Source: CAD feature listing. Evaluate the final solid. Frame: model axes, mm. A direction names the side the tool comes from. Round coordinates to 2 decimals unless told otherwise and drop trailing zeros. Write each loop counter-clockwise with the first axis right and the second up, starting at its lowest first coordinate (ties: lowest second). Pieces come first, ordered by that corner, then holes.
from build123d import *

# Parameters (mm, degrees)
SKETCH1_W           = 40
SKETCH1_H           = 50
BOSS_EXTRUDE1_DEPTH = 10
SKETCH3_W           = 60
SKETCH3_H           = 10
BOSS_EXTRUDE2_DEPTH = 20
FILLET1_R           = 10
SKETCH4_R           = 19.5
SKETCH4_R_2         = 15
BOSS_EXTRUDE3_DEPTH = 20
SKETCH5_R           = 6.5
CUT_EXTRUDE1_DEPTH  = 100


with BuildPart() as part:
    # Sketch1 → Boss-Extrude1 (new body)
    with BuildSketch(Plane.XY):
        Rectangle(SKETCH1_W, SKETCH1_H)
    extrude(amount=BOSS_EXTRUDE1_DEPTH)

    # Sketch3 → Boss-Extrude2 (add, symmetric)
    with BuildSketch(Plane(origin=(0, 0, 0), x_dir=(0, 0, -1), z_dir=(1, 0, 0))):
        with Locations((20, -30)):
            Rectangle(SKETCH3_W, SKETCH3_H)
        with Locations((20, 30)):
            Rectangle(SKETCH3_W, SKETCH3_H)
    extrude(amount=BOSS_EXTRUDE2_DEPTH, both=True)

    # Fillet1
    fillet1_edges = [part.edges().sort_by_distance(p)[0] for p in [
        (0, -35, 10),
        (-20, -30, -50),
        (20, -30, -50),
        (0, 35, 10),
        (-20, 30, -50),
        (20, 30, -50),
    ]]
    fillet(fillet1_edges, radius=FILLET1_R)

    # Sketch4 → Boss-Extrude3 (add)
    with BuildSketch(Plane.XY.offset(10)):
        Circle(SKETCH4_R)
        Circle(SKETCH4_R_2, mode=Mode.SUBTRACT)
    extrude(amount=BOSS_EXTRUDE3_DEPTH)

    # Sketch5 → Cut-Extrude1 (cut)
    with BuildSketch(Plane.XZ.offset(35)):
        with Locations(Location((0, -40, 0), (0, 0, 270))):
            Circle(SKETCH5_R)
    extrude(amount=-CUT_EXTRUDE1_DEPTH, mode=Mode.SUBTRACT)


solid = part.part
1) Section query D-D on x = 16. Return the cut outline in (y, z), then the cut area to 3 significant figures.
Taken from the geometry:
outline: (-35, -48) - (-25, -48) - (-25, 0) - (25, 0) - (25, -48) - (35, -48) - (35, 0) arc R10 ccw to (25, 10) - (11.15, 10) - (11.15, 30) - (-11.15, 30) - (-11.15, 10) - (-25, 10) arc R10 ccw to (-35, 0) - close
area: 2,060 mm2
2) Pull-direction query (X, two-part tool) for faces 4 (the face through (-16.99, 30.07, -47.15)), 5 (the face through (0, -25, -25)), 6 (the face through (0.286, -30.07, -33.506)); classes: released by +X, released by -X, zero draft, split by the parting line, or undercut.
Taken from the geometry:
face 4: released by -X
face 5: zero draft
face 6: undercut
3) Contact query for flat-ended pins moving along their axis: P1, Ø1, axis at x = 1, y = 13, coming from the -Z side; P2, Ø12, axis at x = 6.5, y = -1.5, coming from the +Z side; P3, Ø8, axis at y = -12, z = 22, coming from the -X side. Output: stop coordinate, or through.
Taken from the geometry:
P1: stops at z = 0
P2: stops at z = 10
P3: stops at x = -17.78
4) Section query C-C on y = -4. Return the cut outline in (x, z), then the cut area to 3 significant figures.
Taken from the geometry:
outline: (-20, 0) - (20, 0) - (20, 10) - (19.09, 10) - (19.09, 30) - (14.46, 30) - (14.46, 10) - (-14.46, 10) - (-14.46, 30) - (-19.09, 30) - (-19.09, 10) - (-20, 10) - close
area: 585 mm2
5) Material intervals for line 1 (X direction, y = -32, z = -40); line 2 (Y direction, x = 6.5, z = -43.5); line 3 (Y direction, x = 0, z = 24), sorted ascending.
Taken from the geometry:
line 1: x = -20 to -6.5, 6.5 to 20
line 2: y = -35 to -25, 25 to 35
line 3: y = -19.5 to -15, 15 to 19.5
6) Reachability of faces 1 (the face through (20, 0, 2)), 2 (the face through (0, 0, 0)), 3 (the face through (-2.539, 19.334, 19.86)) from +Z, -Z, +X, -X, +Y, -Y: full face, straight path, thin tool, end or side. Return the list, or none.
Taken from the geometry:
face 1: +Z, -Z, +X, +Y, -Y
face 2: -Z, +X, -X
face 3: +Z
7) Section query A-A on x = 0. Return the cut outline in (y, z).
Taken from the geometry:
outline: (-35, -50) - (-25, -50) - (-25, -46.5) - (-35, -46.5) - close; (-35, -33.5) - (-25, -33.5) - (-25, 0) - (25, 0) - (25, -33.5) - (35, -33.5) - (35, 0) arc R10 ccw to (25, 10) - (19.5, 10) - (19.5, 30) - (15, 30) - (15, 10) - (-15, 10) - (-15, 30) - (-19.5, 30) - (-19.5, 10) - (-25, 10) arc R10 ccw to (-35, 0) - close; (25, -50) - (35, -50) - (35, -46.5) - (25, -46.5) - close
8) Section query B-B on z = -30. Return the cut outline in (x, y).
Taken from the geometry:
outline: (-20, -35) - (20, -35) - (20, -25) - (-20, -25) - close; (-20, 25) - (20, 25) - (20, 35) - (-20, 35) - close
